The listing builds one solid part. Answer for the finished solid, in the listing's coordinates (mm). A direction names the side the tool comes from. Round coordinates to 2 decimals unless told otherwise and drop trailing zeros. Write each loop counter-clockwise with the first axis right and the second up, starting at its lowest first coordinate (ties: lowest second). Pieces come first, ordered by that corner, then holes.
(1) A cutting plane is placed at C-C, the plane x = 49.5. Give the vertices of the cut face in (y, z).
(2) For faces 1 (the face through (80, 0, 0)), 2 (the face through (6.269, -4.336, 19.524)), determine the directions among +Z, -Z, +X, -X, +Y, -Y from which every point of the face is accessible in a straight line to the end or side of a thin tool.
(3) Each of these flat-tipped pins is pushed along its axis until it touches: pin 1 Ø10 at (x, z) = (12, 21) entering from -Y; pin 2 Ø5 at (x, z) = (-23, 2) entering from +Y; pin 3 Ø8 at (x, z) = (35.5, -6) entering from +Y. Where does it stop, or does it pass through?
(4) Find the intervals of material crossed by probe 1 along X at (y, z) = (6.5, 6.5); probe 2 along Z at (x, y) = (-4, -1); probe 3 along X at (y, z) = (-16.5, -26.5), in increasing order.
from build123d import *

# Parameters (mm, degrees)
CHAMFER1_SIZE = 10
CHAMFER2_SIZE = 3


with BuildPart() as part:
    # Sketch1 → Revolve1 (revolve)
    with BuildSketch(Plane.XY):
        Polygon((-80, 0), (-80, 7.5), (-55, 7.5), (-55, 20), (62.928932188, 20), (70, 27.071067812), (70, 40), (80, 40), (80, 0), align=None)
    revolve(axis=Axis((80, 0, 0), (-1, 0, 0)))

    # Chamfer1
    chamfer1_edges = [part.edges().sort_by_distance(p)[0] for p in [
        (80, -40, 0),
    ]]
    chamfer(chamfer1_edges, length=CHAMFER1_SIZE - 0.0001)  # a hair under: the kernel refuses the full size

    # Chamfer2
    chamfer2_edges = [part.edges().sort_by_distance(p)[0] for p in [
        (-55, -20, 0),
    ]]
    chamfer(chamfer2_edges, length=CHAMFER2_SIZE)


solid = part.part
Solutions:
1. outline: circle Ø40 at (0, 0)
2. face 1: +Z, -Z, +X, +Y, -Y
2. face 2: -X
3. pin 1: stops at y = -12
3. pin 2: stops at y = 20
3. pin 3: stops at y = 19.9
4. probe 1: x = -55 to 80
4. probe 2: z = -19.97 to 19.97
4. probe 3: x = 70 to 78.78
